Design review of the part built by this model. Coordinates are the model's own, in mm. Give positions to 0.01 mm unless a question says otherwise; leave off trailing zeros. Loops run counter-clockwise (first coordinate to the right, second up) from the corner with the lowest first, then second, coordinate; pieces in that order, holes last.
from build123d import *

# Parameters (mm, degrees)
F0_R     = 2
F0_R_2   = 4.6
F0_R_3   = 2.5
F1_DEPTH = 1


with BuildPart() as f1:
    # F0 (on Top) → F1 (new body)
    with BuildSketch(Plane.XY):
        with BuildLine():
            Line((-55.638593, -10), (60, -10))
            Line((60, -10), (60, 10))
            Line((60, 10), (-55.638593, 10))
            ThreePointArc((-55.638593, 10), (-87.5, 0), (-55.638593, -10))
        make_face()
        with Locations((-76.505382, -6.505382)):
            Circle(F0_R, mode=Mode.SUBTRACT)
        with Locations((-63.494618, -6.505382)):
            Circle(F0_R, mode=Mode.SUBTRACT)
        with Locations((-70, 0)):
            Circle(F0_R_2, mode=Mode.SUBTRACT)
        with Locations((50, -5)):
            Circle(F0_R_3, mode=Mode.SUBTRACT)
        with Locations((-76.505382, 6.505382)):
            Circle(F0_R, mode=Mode.SUBTRACT)
        with Locations((-63.494618, 6.505382)):
            Circle(F0_R, mode=Mode.SUBTRACT)
        with Locations((50, 5)):
            Circle(F0_R_3, mode=Mode.SUBTRACT)
    extrude(amount=F1_DEPTH)


solid = f1.part
Q1. Wall thickness on line 1 (Y direction, x = 50, z = 0.4); line 2 (X direction, y = -0.5, z = 0.4); line 3 (Y direction, x = -63, z = 0.6): over which ranges is each line inside the solid? List them lowest first.
Results:
line 1: y = -10 to -7.5, -2.5 to 2.5, 7.5 to 10
line 2: x = -87.49 to -74.57, -65.43 to 60
line 3: y = -16.04 to -8.44, -4.57 to 4.57, 8.44 to 16.04
Q2. Take a section at D-D (z = 0.35). Give the boundary of the cut face in (x, y).
Results:
outline: (-55.64, -10) - (60, -10) - (60, 10) - (-55.64, 10) arc R17.5 ccw (long way) to start; hole circle Ø4 at (-76.51, -6.51); hole circle Ø4 at (-76.51, 6.51); hole circle Ø9.2 at (-70, 0); hole circle Ø4 at (-63.49, -6.51); hole circle Ø4 at (-63.49, 6.51); hole circle Ø5 at (50, -5); hole circle Ø5 at (50, 5)
Q3. Take a section at B-B (y = 0). Give the boundary of the cut face in (x, z).
Results:
outline: (-87.5, 0) - (-74.6, 0) - (-74.6, 1) - (-87.5, 1) - close; (-65.4, 0) - (60, 0) - (60, 1) - (-65.4, 1) - close
Q4. Draft analysis for pull direction X (two halves, no side actions). For faces 1 (the face through (-15, 0, 1)), 2 (the face through (-87.49, 0.62, 0.49)), 3 (the face through (-74.596, 0.202, 0.493)), state which applies: pulls with the +X half, pulls with the -X half, needs draft (parallel to the pull), parting line crosses it, or undercut.
Results:
face 1: needs draft
face 2: parting line crosses it
face 3: undercut
Q5. Take a section at C-C (x = 50). Give the boundary of the cut face in (y, z).
Results:
outline: (-10, 0) - (-7.5, 0) - (-7.5, 1) - (-10, 1) - close; (-2.5, 0) - (2.5, 0) - (2.5, 1) - (-2.5, 1) - close; (7.5, 0) - (10, 0) - (10, 1) - (7.5, 1) - close
Q6. Take a section at A-A (x = -70). Give the boundary of the cut face in (y, z), plus the area to 3 significant figures.
Results:
outline: (-17.5, 0) - (-4.6, 0) - (-4.6, 1) - (-17.5, 1) - close; (4.6, 0) - (17.5, 0) - (17.5, 1) - (4.6, 1) - close
area: 25.8 mm2
